Autodesk Inventor part; units mm, degrees
ref_plane "Work Plane1" through (0, -31.75, 0) normal (0, 1, 0) x (-1, 0, 0)
ref_plane "YZ Plane" through (0, 0, 0) normal (1, 0, 0) x (0, 1, 0)
ref_plane "XZ Plane" through (0, 0, 0) normal (0, 1, 0) x (-1, 0, 0)
sketch "Sketch2" plane through (0, 0, 0) normal (0, 0, 1) x (1, 0, 0)
  line L0 (-31.75, 50.8) -> (31.75, 50.8)
  line L1 (34.925, 47.625) -> (34.925, -47.625)
  line L2 (31.75, -50.8) -> (-31.75, -50.8)
  line L3 (-34.925, -47.625) -> (-34.925, 47.625)
  arc A0 (-31.75, 50.8) -> (-34.925, 47.625) centre (-31.75, 47.625) ccw
  arc A1 (34.925, 47.625) -> (31.75, 50.8) centre (31.75, 47.625) ccw
  arc A2 (31.75, -50.8) -> (34.925, -47.625) centre (31.75, -47.625) ccw
  arc A3 (-34.925, -47.625) -> (-31.75, -50.8) centre (-31.75, -47.625) ccw
  point P0 (0, 0)
  point P1 (-34.925, 50.8)
  point P2 (34.925, -50.8)
  point P3 (34.925, 50.8)
  point P4 (-34.925, -50.8)
  point P5 (-34.925, 0)
  point P6 (0, 50.8)
  dimension "d0" = 69.85
  dimension "d1" = 101.6
  dimension "d4" = 3.175
extrude "Extrusion1" add sketch "Sketch2" along normal blind 1.524
sketch "Sketch3" plane through (0, 0, 1.524) normal (0, 0, 1) x (1, 0, 0)
  line L0 (-19.05, 38.1) -> (19.05, 38.1)
  line L1 (22.225, 34.925) -> (22.225, -34.925)
  line L2 (19.05, -38.1) -> (-19.05, -38.1)
  line L3 (-22.225, -34.925) -> (-22.225, 34.925)
  arc A0 (-19.05, 38.1) -> (-22.225, 34.925) centre (-19.05, 34.925) ccw
  arc A1 (22.225, 34.925) -> (19.05, 38.1) centre (19.05, 34.925) ccw
  arc A2 (19.05, -38.1) -> (22.225, -34.925) centre (19.05, -34.925) ccw
  arc A3 (-22.225, -34.925) -> (-19.05, -38.1) centre (-19.05, -34.925) ccw
  line L4 (31.75, -50.8) -> (-31.75, -50.8)
  line L5 (-34.925, -47.625) -> (-34.925, 47.625)
  point P0 (0, 0)
  point P1 (0, 38.1)
  point P2 (-22.225, 0)
  dimension "d7" = 3.175
  dimension "d8" = 12.7
  dimension "d9" = 12.7
extrude "Extrusion2" add sketch "Sketch3" along normal blind 6.35
fillet "Fillet1" radius 3.175 16 edges at (0, 38.1, 7.874) (21.2951, 37.1701, 7.874) (22.225, 0, 7.874) (21.2951, -37.1701, 7.874) (0, -38.1, 7.874) (-21.2951, -37.1701, 7.874) (-22.225, 0, 7.874) (-21.2951, 37.1701, 7.874) (0, 38.1, 1.524) (21.2951, 37.1701, 1.524) (22.225, 0, 1.524) (21.2951, -37.1701, 1.524) (0, -38.1, 1.524) (-21.2951, -37.1701, 1.524) (-22.225, 0, 1.524) (-21.2951, 37.1701, 1.524)
ref_plane "Work Plane1" through (0, -31.75, 0) normal (0, 1, 0) x (-1, 0, 0)
sketch "Sketch4" plane through (0, -31.75, 0) normal (0, 1, 0) x (-1, 0, 0)
  line L0 (-15.875, 0) -> (15.875, 0)
  line L1 (15.875, 0) -> (15.875, 25.4)
  line L2 (15.875, 25.4) -> (-15.875, 25.4)
  line L3 (-15.875, 25.4) -> (-15.875, 0)
  circle A0 centre (0, 25.4) radius 15.875
  line L4 (-31.75, 0) -> (31.75, 0)
  point P0 (0, 0)
  point P1 (0, 0)
  point P2 (0, 0)
  dimension "d15" = 31.75
  dimension "d14" = 25.4
extrude "Extrusion3" add sketch "Sketch4" against normal blind 1.524
mirror "Mirror1" about plane through (0, 0, 0) normal (0, 1, 0) of "Extrusion3"
sketch "Sketch5" plane through (0, 0, 1.524) normal (0, 0, 1) x (1, 0, 0)
  circle A0 centre (-28.575, -44.45) radius 2.54
  line L0 (-34.925, -47.625) -> (-34.925, 47.625)
  line L1 (31.75, -50.8) -> (-31.75, -50.8)
  point P0 (0, 0)
  dimension "d18" = 5.08
  dimension "d19" = 6.35
  dimension "d20" = 6.35
extrude "Extrusion4" cut sketch "Sketch5" against normal through all
mirror "Mirror2" about plane through (0, 0, 0) normal (0, 1, 0) of "Extrusion4"
mirror "Mirror3" about plane through (0, 0, 0) normal (1, 0, 0) of "Extrusion4", "Mirror2"
Read the model definition and answer for the solid it produces. Units are mm, in the model's axes. A direction names the side the tool comes from. Round coordinates to 2 decimals unless told otherwise and drop trailing zeros. Write each loop counter-clockwise with the first axis right and the second up, starting at its lowest first coordinate (ties: lowest second). Pieces come first, ordered by that corner, then holes. Notation, with made-up numbers: (-25, -33) - (6, -33) arc R33 ccw to (6, 4) - close; hole circle Ø10 at (-33, -14). An arc over 180 degrees is marked (long way). One line per item, written item: value.
Q1. Straight lines are drawn through the part: line 1 (Y direction, x = -4, z = 35.5); line 2 (Z direction, x = -5.5, y = 42); line 3 (Z direction, x = -7, y = -3). For each, find the intervals that lie inside material, in ascending order. Write a range as from..to.
The answers:
line 1: y = -33.27..-31.75, 31.75..33.27
line 2: z = 0..1.52
line 3: z = 0..7.87
Q2. Which of the six approach directions +Z, -Z, +X, -X, +Y, -Y give full straight-line access (tool end or side, diameter ignored) to faces 4 (the cylindrical face through (0.267, 39.005, 2.479)), 5 (the flat face through (0, 31.75, 25)), 6 (the flat face through (0, -33.274, 25))?
The answers:
face 4: +Z, +X, -X, +Y
face 5: +Z, +X, -X
face 6: +Z, +X, -X, -Y
Q3. Find section B-B (z = 14.5). Determine the outline of the cut face in (x, y) (3 decimals), and give its area (3 significant figures).
The answers:
outline: (-15.875, -33.274) - (15.875, -33.274) - (15.875, -31.75) - (-15.875, -31.75) - close; (-15.875, 31.75) - (15.875, 31.75) - (15.875, 33.274) - (-15.875, 33.274) - close
area: 96.8 mm2
Q4. Each of these flat-tipped pins is pushed along its axis until it touches: P1, Ø4, axis at x = 22.5, y = -0.5, coming from the +Z side; P2, Ø10, axis at x = 10, y = 0.5, coming from the +Z side; P3, Ø5, axis at x = -19, z = 32, coming from the +Y side; P4, Ø4, axis at x = -7, z = 17.5, coming from the -Y side. Where does it stop, or does it pass through?
The answers:
P1: stops at z = 7.52
P2: stops at z = 7.87
P3: passes through
P4: stops at y = -33.27
Q5. For a pull along X with two mould halves and no side action, classify faces 1 (the cylindrical face through (34.02, -49.845, 0.751)), 2 (the cylindrical face through (-0.267, -37.195, 6.919)), 3 (the cylindrical face through (26.229, 45.423, 0.773)) as pulls with the +X half, pulls with the -X half, needs draft (parallel to the pull), parting line crosses it, or undercut.
The answers:
face 1: pulls with the +X half
face 2: needs draft
face 3: undercut
Q6. Find section C-C (x = 30). Determine the outline of the cut face in (y, z), and give its area (3 significant figures).
The answers:
outline: (-50.8, 0) - (-46.55, 0) - (-46.55, 1.52) - (-50.8, 1.52) - close; (-42.35, 0) - (42.35, 0) - (42.35, 1.52) - (-42.35, 1.52) - close; (46.55, 0) - (50.8, 0) - (50.8, 1.52) - (46.55, 1.52) - close
area: 142 mm2
Q7. Find section A-A (y = 44.45). Determine the outline of the cut face in (x, z) (3 decimals), and give its area (3 significant figures).
The answers:
outline: (-34.925, 0) - (-31.115, 0) - (-31.115, 1.524) - (-34.925, 1.524) - close; (-26.035, 0) - (26.035, 0) - (26.035, 1.524) - (-26.035, 1.524) - close; (31.115, 0) - (34.925, 0) - (34.925, 1.524) - (31.115, 1.524) - close
area: 91.0 mm2
